Work out the finished part from the listing and answer in its coordinate system (mm). Face numbers are marked on the shaded views. Round coordinates to 2 decimals unless told otherwise and drop trailing zeros. Order: outer loops, then holes, each group sorted by start corner. A loop starts at its lowest first (then second) coordinate and runs counter-clockwise, first axis right, second up.
from build123d import *

# Parameters (mm, degrees)
F1_DEPTH = 10


with BuildPart() as f1:
    # F0 (on Front) → F1 (new body)
    with BuildSketch(Plane.XZ):
        with BuildLine():
            Line((25, -25.975256), (25, 0))
            ThreePointArc((25, 0), (0, -25), (-25, 0))
            Line((-25, 0), (-25, -25.975256))
            Line((-25, -25.975256), (25, -25.975256))
        make_face()
        with BuildLine():
            Line((2.5, 0), (25, 0))
            ThreePointArc((25, 0), (0, 25), (-25, 0))
            Line((-25, 0), (-2.5, 0))
            ThreePointArc((-2.5, 0), (0, 2.5), (2.5, 0))
        make_face()
        with BuildLine():
            ThreePointArc((-25, 0), (0, -25), (25, 0))
            Line((25, 0), (2.5, 0))
            ThreePointArc((2.5, 0), (0, -2.5), (-2.5, 0))
            Line((-2.5, 0), (-25, 0))
        make_face()
    extrude(amount=F1_DEPTH)


solid = f1.part
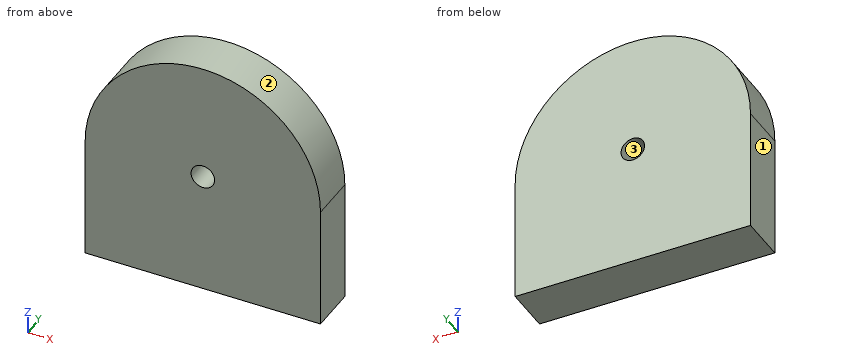
Item 1: Find section C-C (x = 7). Write down the section's boundary in (y, z), plus the area to 3 significant figures.
Item 2: Find section B-B (y = -1). Write down the section's boundary in (x, z).
Item 3: Find section D-D (z = 5). Write down the section's boundary in (x, y).
Item 4: Given pin 1 (6 mm diameter, centred on x = 11.5, y = -6, fed in from +Z), flat-ended and moving along its own axis, determine where the tip first touches the part or whether it passes through.
Item 5: Find the intervals of material crossed by line 1 along Z through (x, y) = (0, -6); line 2 along Z through (x, y) = (-2, -0.25); line 3 along X through (y, z) = (-4, 19), in increasing order.
Item 6: For a pull along Z with two mould halves and no side action, classify the marked faces 1, 2 and 3 as released by +Z, released by -Z, zero draft, split by the parting line, or undercut.
Item 7: Find section A-A (x = 0). Write down the section's boundary in (y, z), plus the area to 3 significant figures.
Model answer:
1. outline: (-10, -25.98) - (0, -25.98) - (0, 24) - (-10, 24) - close
1. area: 500 mm2
2. outline: (-25, -25.98) - (25, -25.98) - (25, 0) arc R25 ccw to (-25, 0) - close; hole circle Ø5 at (0, 0)
3. outline: (-24.49, -10) - (24.49, -10) - (24.49, 0) - (-24.49, 0) - close
4. pin 1: stops at z = 23.51
5. line 1: z = -25.98 to -2.5, 2.5 to 25
5. line 2: z = -25.98 to -1.5, 1.5 to 24.92
5. line 3: x = -16.25 to 16.25
6. face 1: zero draft
6. face 2: released by +Z
6. face 3: undercut
7. outline: (-10, -25.98) - (0, -25.98) - (0, -2.5) - (-10, -2.5) - close; (-10, 2.5) - (0, 2.5) - (0, 25) - (-10, 25) - close
7. area: 460 mm2
